Input: dimensioned drawing with shaded views. Units: mm. Origin: part minimum x, y, z. A direction names the side the tool comes from. Coordinates: 2 decimals unless noted, no trailing zeros. Order: outer loops, then holes, each group sorted by start corner. A loop starts at its lowest first (then second) coordinate and runs counter-clockwise, first axis right, second up. Notation, with made-up numbers: (27, -40) -> (51, -40) arc R34 ccw to (51, -10) -> close; hole circle Ø6 at (57.25, 69.5). An arc over 180 degrees is marked (long way). Put each result on its own line as item: value.
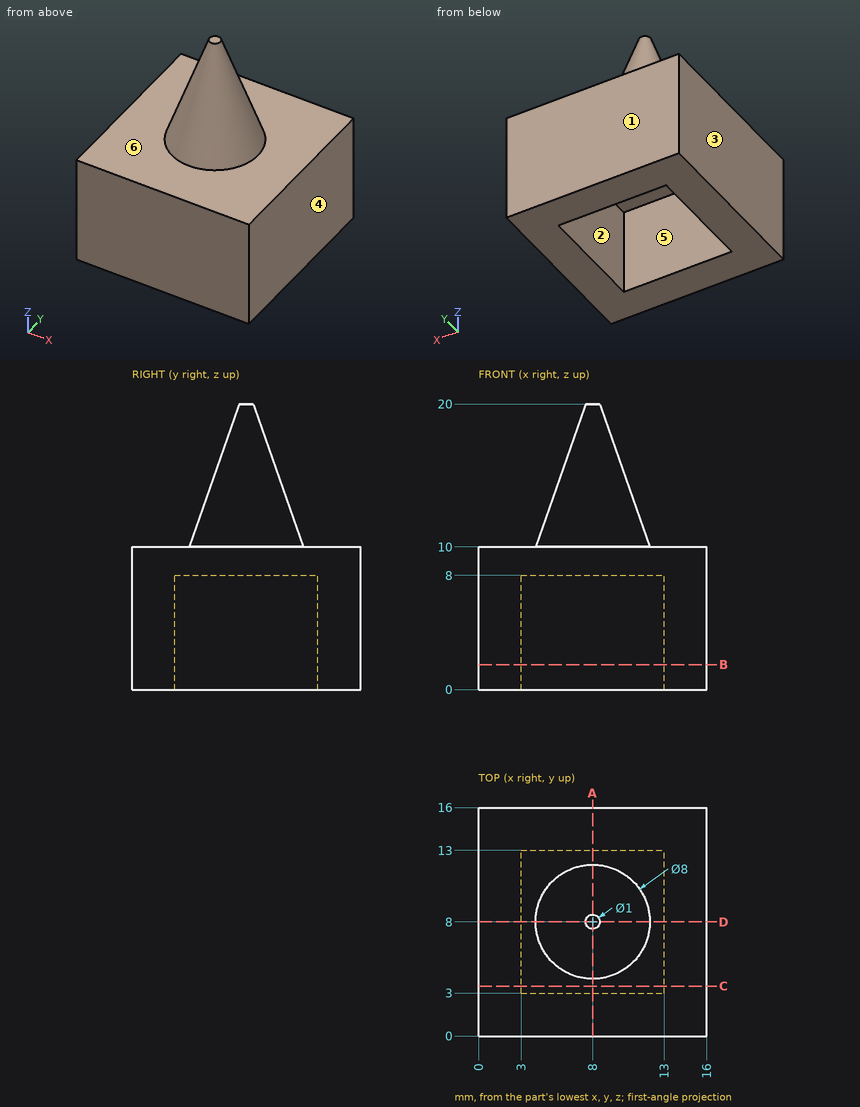
1. Cut plane B-B on z = 1.75. Output: boundary loops of the cut face in (x, y), plus the area to 3 significant figures.
Numbers:
outline: (0, 0) -> (16, 0) -> (16, 16) -> (0, 16) -> close; hole (3, 3) -> (13, 3) -> (13, 13) -> (3, 13) -> close
area: 156 mm2
2. First-contact query: pin 1 (5 mm diameter, centred on x = 5.5, z = 10.5, fed in from +Y); pin 2 (2 mm diameter, centred on x = 11, y = 11, fed in from -Z); pin 3 (1 mm diameter, centred on x = 6.5, y = 3, fed in from +Z). Flat tips, straight axial feed; report the tip coordinate or a pass-through.
Numbers:
pin 1: stops at y = 16
pin 2: stops at z = 8
pin 3: stops at z = 10
3. Ray query, line 1 along X through (y, z) = (10.75, 5.5); line 2 along Z through (x, y) = (6, 11.75). Return the intervals inside material, ascending.
Numbers:
line 1: x = 0 to 3, 13 to 16
line 2: z = 8 to 10
4. Pull-direction query (Y, two-part tool) for the marked faces 1, 2 and 3; classes: pulls with the +Y half, pulls with the -Y half, needs draft (parallel to the pull), parting line crosses it, or undercut.
Numbers:
face 1: pulls with the +Y half
face 2: undercut
face 3: needs draft
5. Cut plane C-C on y = 3.5. Output: boundary loops of the cut face in (x, z), plus the area to 3 significant figures.
Numbers:
outline: (0, 0) -> (3, 0) -> (3, 8) -> (13, 8) -> (13, 0) -> (16, 0) -> (16, 10) -> (0, 10) -> close
area: 80.0 mm2
6. Set-up query: the marked faces 4, 5 and 6. Return all of +Z, -Z, +X, -X, +Y, -Y with unobstructed straight access to the full face (end or side cutting, diameter ignored); none if empty.
Numbers:
face 4: +Z, -Z, +X, +Y, -Y
face 5: -Z
face 6: +Z
7. Cut plane A-A on x = 8. Output: boundary loops of the cut face in (y, z), plus the area to 3 significant figures.
Numbers:
outline: (0, 0) -> (3, 0) -> (3, 8) -> (13, 8) -> (13, 0) -> (16, 0) -> (16, 10) -> (12, 10) -> (8.5, 20) -> (7.5, 20) -> (4, 10) -> (0, 10) -> close
area: 125 mm2
